```python
from build123d import *

# Parameters (mm, degrees)
BOSS_EXTRUDE1_DEPTH = 44.45
CUT_EXTRUDE1_DEPTH  = 7.35


with BuildPart() as part:
    # Sketch3 → Boss-Extrude1 (new body, symmetric)
    with BuildSketch(Plane(origin=(0, 0, 0), x_dir=(0, 0, -1), z_dir=(1, 0, 0))):
        Polygon((-88.825470595, 3.175), (-85.159296386, -3.175), (60.083377372, -3.175), (71.0819, 3.175), align=None)
    extrude(amount=BOSS_EXTRUDE1_DEPTH, both=True)

    # Sketch5 → Cut-Extrude1 (cut, through all)
    with BuildSketch(Plane(origin=(0, 3.175, 0), x_dir=(1, 0, 0), z_dir=(0, 1, 0))):
        with BuildLine():
            ThreePointArc((-31.75, 71.0819), (0, 39.3319), (31.75, 71.0819))
            Line((31.75, 71.0819), (-31.75, 71.0819))
        make_face()
    extrude(amount=-CUT_EXTRUDE1_DEPTH, mode=Mode.SUBTRACT)


solid = part.part
```
Input: part model. Units: mm. Frame: model coordinates. Coordinates: 2 decimals unless noted, no trailing zeros. Write each loop counter-clockwise with the first axis right and the second up, starting at its lowest first coordinate (ties: lowest second). Pieces come first, ordered by that corner, then holes. Notation, with made-up numbers: (39.5, 9) -> (88.5, 9) arc R26 ccw to (88.5, 33) -> close; hole circle Ø3 at (-20.5, 34.5). An arc over 180 degrees is marked (long way). Write each question's results on one line, items separated by ' | '.
Item 1: Material intervals for probe 1 along X at (y, z) = (-1.5, -49); probe 2 along Z at (x, y) = (17.5, 1); probe 3 along Z at (x, y) = (-22, -1.75), sorted ascending.
Conclusion:
probe 1: x = -44.45 to -22.81, 22.81 to 44.45 | probe 2: z = -44.59 to 87.57 | probe 3: z = -48.19 to 85.98
Item 2: Section query B-B on y = 1. Return loops of the section in (x, z), plus the area to 3 significant figures.
Conclusion:
outline: (-44.45, -67.31) -> (-31.53, -67.31) arc R31.75 cw to (31.53, -67.31) -> (44.45, -67.31) -> (44.45, 87.57) -> (-44.45, 87.57) -> close | area: 12,400 mm^2
Item 3: Section query A-A on x = -36. Return loops of the section in (y, z) (3 decimals).
Conclusion:
outline: (-3.175, -60.083) -> (3.175, -71.082) -> (3.175, 88.825) -> (-3.175, 85.159) -> close
Item 4: Section query C-C on x = 0. Return loops of the section in (y, z) (3 decimals).
Conclusion:
outline: (-3.175, -39.332) -> (3.175, -39.332) -> (3.175, 88.825) -> (-3.175, 85.159) -> close
